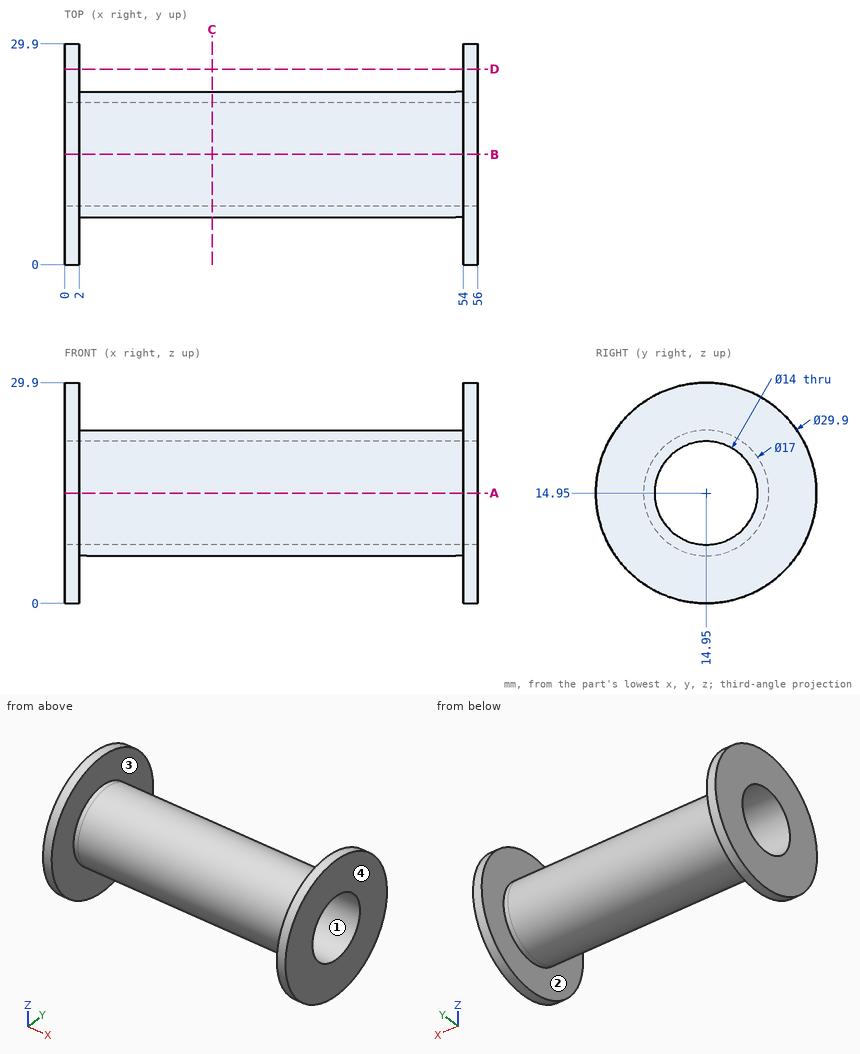
Answer from the drawing. Dimensions are ordinates in mm from the lowest x, y and z of the part. A direction names the side the tool comes from. Round coordinates to 2 decimals unless told otherwise and drop trailing zeros. Loops run counter-clockwise (first coordinate to the right, second up) from the corner with the lowest first, then second, coordinate; pieces in that order, holes last. Notation, with made-up numbers: (63.5, 7) - (100.5, 7) arc R18 ccw to (100.5, 11) - close; hole circle Ø7 at (80.5, 75.25). An arc over 180 degrees is marked (long way). Return JSON: item names as keys, results as strings. Group by question number.
1. Each of these flat-tipped pins is pushed along its axis until it touches: P1, Ø6, axis at x = 28, z = 13.5, coming from the +Y side; P2, Ø1.5, axis at x = 10, z = 12.5, coming from the +Y side; P3, Ø5, axis at x = 50, y = 7, coming from the +Z side; P4, Ø12.5, axis at y = 14.95, z = 14.95, coming from the -X side. Where does it stop, or does it pass through?
2. The part is cut by section D-D on y = 26.5. Determine the outline of the cut face in (x, z), then the cut area to 3 significant figures.
3. Which of the six approach directions +Z, -Z, +X, -X, +Y, -Y give full straight-line access (tool end or side, diameter ignored) to the marked faces 3 and 4?
4. Consider probe 1 along Y at (x, z) = (36.5, 14.95); probe 2 along X at (y, z) = (24.75, 5.5). Determine where each line is inside the solid, lowest interval first.
5. The part is cut by section C-C on x = 20. Determine the outline of the cut face in (y, z).
6. The mould has two halves that part along Y. Classify the marked faces 1 and 2: pulls with the +Y half, pulls with the -Y half, needs draft (parallel to the pull), parting line crosses it, or undercut.
7. The part is cut by section A-A on z = 14.95. Determine the outline of the cut face in (x, y).
Resolved:
{
 "1": {"P1": "stops at y = 23.45", "P2": "stops at y = 23.28", "P3": "stops at z = 21.47", "P4": "passes through"},
 "2": {"outline": "(0, 5.46) - (2, 5.46) - (2, 24.44) - (0, 24.44) - close; (54, 5.46) - (56, 5.46) - (56, 24.44) - (54, 24.44) - close", "area": "75.9 mm²"},
 "3": {"face 3": "none", "face 4": "+Z, -Z, +X, +Y, -Y"},
 "4": {"probe 1": "y = 6.45 to 7.95, 21.95 to 23.45", "probe 2": "x = 0 to 2, 54 to 56"},
 "5": {"outline": "circle Ø17 at (14.95, 14.95); hole circle Ø14 at (14.95, 14.95)"},
 "6": {"face 1": "undercut", "face 2": "needs draft"},
 "7": {"outline": "(0, 0) - (2, 0) - (2, 6.45) - (54, 6.45) - (54, 0) - (56, 0) - (56, 7.95) - (0, 7.95) - close; (0, 21.95) - (56, 21.95) - (56, 29.9) - (54, 29.9) - (54, 23.45) - (2, 23.45) - (2, 29.9) - (0, 29.9) - close"}
}
